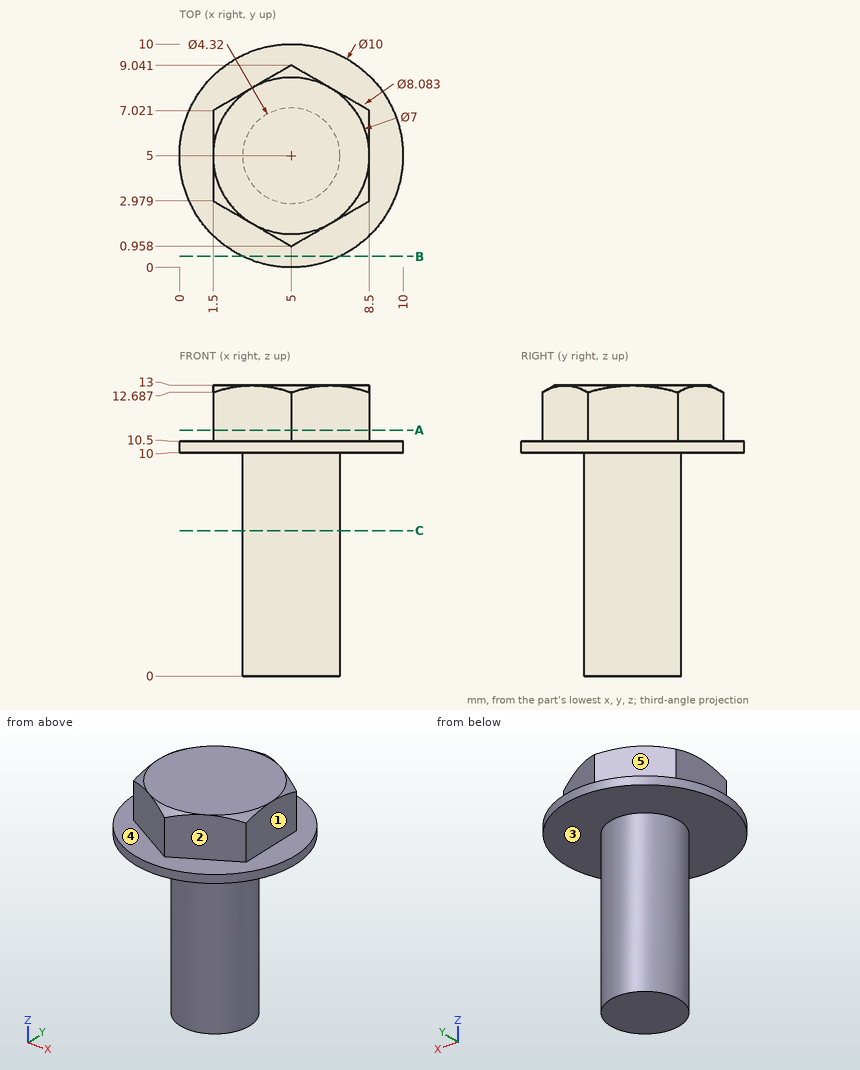
Print and shaded views of the part. All mm, measured from the part's lowest x, y and z. A direction names the side the tool comes from. Give positions to 0.01 mm unless a question says otherwise; leave off trailing zeros. Loops run counter-clockwise (first coordinate to the right, second up) from the corner with the lowest first, then second, coordinate; pieces in that order, holes last.
1) Flat gauge pins, fed straight in: pin 1 Ø4 at (y, z) = (8, 2.5) entering from +X (1 decimal); pin 2 Ø1.2 at (y, z) = (6, 12) entering from -X; pin 3 Ø4 at (y, z) = (8.5, 2) entering from -X (1 decimal); pin 4 Ø1.5 at (x, z) = (1, 5.5) entering from -Y. Where does each tip first touch, or does it go through?
2) Saw through at B-B (y = 0.5). Write the cut outline in (x, z).
3) Wall check: line 1 (X direction, y = 4.25, z = 3) (1 decimal); line 2 (Z direction, x = 3.5, y = 7.5); line 3 (Z direction, x = 8.5, y = 1.75). Give the ranges that are in metal, low to high.
4) Saw through at C-C (z = 6.5). Write the cut outline in (x, y).
5) Saw through at A-A (z = 11). Write the cut outline in (x, y).
6) Tool access for the marked faces 1, 2, 3, 4 and 5: list every direction of +Z, -Z, +X, -X, +Y, -Y with a clear straight run to the whole face (end or side of a thin tool).
Answer block:
1. pin 1: stops at x = 6.9
1. pin 2: stops at x = 1.5
1. pin 3: stops at x = 3.4
1. pin 4: passes through
2. outline: (2.82, 10) - (7.18, 10) - (7.18, 10.5) - (2.82, 10.5) - close
3. line 1: x = 3 to 7
3. line 2: z = 10 to 13
3. line 3: z = 10 to 10.5
4. outline: circle Ø4.32 at (5, 5)
5. outline: (1.5, 2.98) - (5, 0.96) - (8.5, 2.98) - (8.5, 7.02) - (5, 9.04) - (1.5, 7.02) - close
6. face 1: +Z, +X, +Y, -Y
6. face 2: +Z, +X, -Y
6. face 3: -Z
6. face 4: +Z
6. face 5: +Z, -X, +Y
